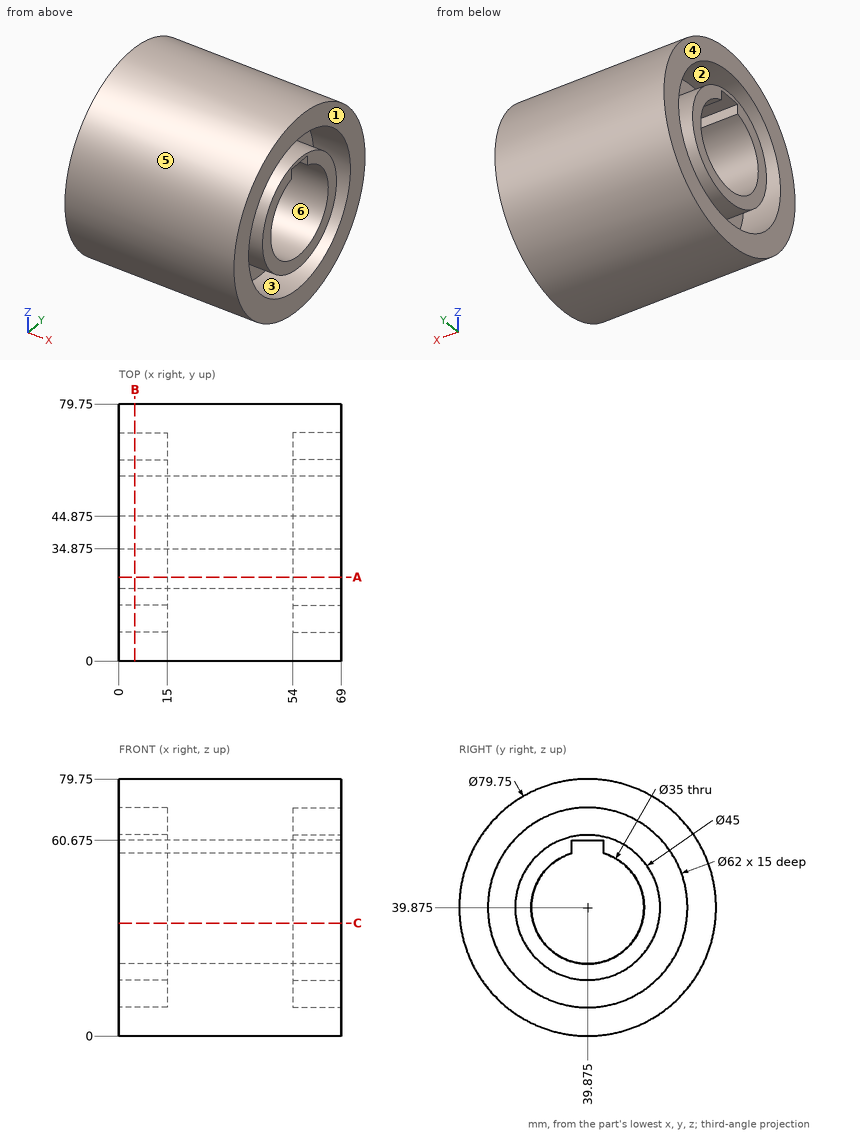
Study the drawing (mm; zero at the part's minimum x, y, z) and answer. A direction names the side the tool comes from. Coordinates: 2 decimals unless noted, no trailing zeros. Loops run counter-clockwise (first coordinate to the right, second up) from the corner with the lowest first, then second, coordinate; pieces in that order, holes last. Notation, with made-up numbers: (32, 27) -> (87, 27) arc R11 ccw to (87, 45) -> close; hole circle Ø9 at (55, 55). An arc over 180 degrees is marked (long way). Write each question's results on one line, items separated by ' | '. Start each with the question number.
1) Find section A-A on y = 26. Determine the outline of the cut face in (x, z), then the cut area to 3 significant figures.
2) Consider line 1 along Y through (x, z) = (63, 46); line 2 along Z through (x, y) = (4, 37) (3 decimals); line 3 along Y through (x, z) = (65, 44). Determine where each line is inside the solid, lowest interval first.
3) Find section C-C on z = 35. Determine the outline of the cut face in (x, y), then the cut area to 3 significant figures.
4) Flat-ended cylindrical pins translate along their axes: P1, Ø10, axis at y = 63, z = 70.5, coming from the -X side; P2, Ø3, axis at x = 27, z = 58.5, coming from the +Y side; P3, Ø2, axis at x = 42.5, z = 23, coming from the -Y side; P4, Ø5, axis at x = 28, y = 39, coming from the -Z side. Find the tip coordinate at first contact, or state that the pin passes through.
5) The mould has two halves that part along Y. Classify the marked faces 4, 5 and 6: pulls with the +Y half, pulls with the -Y half, needs draft (parallel to the pull), parting line crosses it, or undercut.
6) For the marked faces 1, 2 and 3, determine the directions among +Z, -Z, +X, -X, +Y, -Y from which every point of the face is accessible in a straight line to the end or side of a thin tool.
7) Find section B-B on x = 5. Count the separate pieces of the cut face and the enclosed holes in it, then the cut area to 3 significant figures.
Response values:
1) outline: (0, 2.49) -> (69, 2.49) -> (69, 12.15) -> (54, 12.15) -> (54, 22.16) -> (69, 22.16) -> (69, 29.21) -> (0, 29.21) -> (0, 22.16) -> (15, 22.16) -> (15, 12.15) -> (0, 12.15) -> close; (0, 50.54) -> (69, 50.54) -> (69, 57.59) -> (54, 57.59) -> (54, 67.6) -> (69, 67.6) -> (69, 77.26) -> (0, 77.26) -> (0, 67.6) -> (15, 67.6) -> (15, 57.59) -> (0, 57.59) -> close | area: 3,090 mm^2
2) line 1: y = 0.47 to 9.49, 18.22 to 23.48, 56.27 to 61.53, 70.26 to 79.28 | line 2: z = 0.104 to 9.009, 17.559 to 22.613, 60.675 to 62.191, 70.741 to 79.646 | line 3: y = 0.21 to 9.15, 17.76 to 22.87, 56.88 to 61.99, 70.6 to 79.54
3) outline: (0, 0.3) -> (69, 0.3) -> (69, 9.26) -> (54, 9.26) -> (54, 17.91) -> (69, 17.91) -> (69, 23.07) -> (0, 23.07) -> (0, 17.91) -> (15, 17.91) -> (15, 9.26) -> (0, 9.26) -> close; (0, 56.68) -> (69, 56.68) -> (69, 61.84) -> (54, 61.84) -> (54, 70.49) -> (69, 70.49) -> (69, 79.45) -> (0, 79.45) -> (0, 70.49) -> (15, 70.49) -> (15, 61.84) -> (0, 61.84) -> close | area: 2,620 mm^2
4) P1: stops at x = 0 | P2: stops at y = 75.89 | P3: stops at y = 3.3 | P4: stops at z = 0
5) face 4: needs draft | face 5: parting line crosses it | face 6: undercut
6) face 1: +Z, -Z, +X, +Y, -Y | face 2: -X | face 3: +X
7) separate pieces: 2 | enclosed holes: 2 | area: 2,570 mm^2
